```python
from build123d import *

# Parameters (mm, degrees)
F0_W     = 35.2
F0_H     = 35.2
F0_W_2   = 26
F0_H_2   = 26
F0_R     = 11
F0_R_2   = 2.5
F1_DEPTH = 42
F2_DEPTH = 2
F3_DEPTH = 25
F4_R     = 3
F5_D     = 3
F5_DEPTH = 5
F5_TIP   = 0.9012909285


with BuildPart() as f1:
    # F0 (on Top) → F1 (new body)
    with BuildSketch(Plane.XY):
        Rectangle(F0_W, F0_H)
        Rectangle(F0_W_2, F0_H_2, mode=Mode.SUBTRACT)
        Rectangle(F0_W_2, F0_H_2)
        Circle(F0_R, mode=Mode.SUBTRACT)
        Circle(F0_R)
        Circle(F0_R_2, mode=Mode.SUBTRACT)
        Circle(F0_R_2)
    extrude(amount=-F1_DEPTH)

    # F0 (on Top) → F2 (join)
    with BuildSketch(Plane.XY):
        Circle(F0_R)
        Circle(F0_R_2, mode=Mode.SUBTRACT)
    extrude(amount=F2_DEPTH)

    # F0 (on Top) → F3 (join)
    with BuildSketch(Plane.XY):
        Circle(F0_R_2)
    extrude(amount=F3_DEPTH)

    # F4
    f4_edges = [f1.edges().sort_by_distance(p)[0] for p in [
        (17.6, 17.6, -21),
        (17.6, -17.6, -21),
        (-17.6, -17.6, -21),
        (-17.6, 17.6, -21),
    ]]
    fillet(f4_edges, radius=F4_R)

    # F5
    with Locations(Plane.XY):
        with Locations((-13, 13), (13, 13), (13, -13), (-13, -13)):
            Hole(F5_D / 2, depth=F5_DEPTH)
            with Locations((0, 0, -(F5_DEPTH + F5_TIP / 2))):  # 118° drill point
                Cone(0, F5_D / 2, F5_TIP, mode=Mode.SUBTRACT)


solid = f1.part
```
The model under review builds one solid part; all positions refer to its coordinate system, in mm. A direction names the side the tool comes from. Coordinates: 2 decimals unless noted, no trailing zeros. Write each loop counter-clockwise with the first axis right and the second up, starting at its lowest first coordinate (ties: lowest second). Pieces come first, ordered by that corner, then holes. Notation, with made-up numbers: (59.5, -31) -> (83.5, -31) arc R29 ccw to (83.5, -10) -> close; hole circle Ø6 at (8, 43.25). An arc over 180 degrees is marked (long way). One line per item, written item: value. Start each with the question number.
Q1. Clearance check with flat-ended pins moving along their axes: P1, Ø2.5, axis at x = -13, y = -13, coming from the +Z side; P2, Ø8, axis at x = 4, y = -9.5, coming from the +Z side; P3, Ø4, axis at x = -1.5, z = 3.5, coming from the +Y side. State where each tip first meets the part, or that it passes through.
Q2. Add section C-C, the plane x = -9.5. Give the boundary of the cut face in (y, z), then the cut area to 3 significant figures.
Q3. The part is to be moulded in two halves that separate along X. For faces 1 (the face through (-2.38, -10.74, 0.99)), 2 (the face through (-11.5, 13.07, -2.54)), 3 (the face through (14.5, 13.07, -2.54)), 4 (the face through (-16.74, 16.7, -21.29)), say which applies: +X half, -X half, draft (parallel to the pull), parting line (faces both ways), or undercut.
Q4. To check wall thickness, follow probe 1 along Y at (x, z) = (13, -2.85); probe 2 along Z at (x, y) = (-6.5, -14). State the ranges of each line that lie inside material, in increasing order.
Q5. Add section A-A, the plane x = 0. Give the boundary of the cut face in (y, z).
Q6. Add section D-D, the plane y = 7. Give the boundary of the cut face in (x, z).
Q7. For faces 5 (the face through (14.5, -12.93, -2.54)), 6 (the face through (0, 0, -42)), list the 3-axis set-ups (+Z, -Z, +X, -X, +Y, -Y) from which the entire face can be reached by the end or side of a thin tool; tool diameter is ignored.
Response:
1. P1: z = -5.15
1. P2: z = 2
1. P3: y = 11
2. outline: (-17.6, -42) -> (17.6, -42) -> (17.6, 0) -> (5.55, 0) -> (5.55, 2) -> (-5.55, 2) -> (-5.55, 0) -> (-17.6, 0) -> close
2. area: 1,500 mm²
3. face 1: parting line
3. face 2: undercut
3. face 3: undercut
3. face 4: -X half
4. probe 1: -17.6 to -14.5, -11.5 to 11.5, 14.5 to 17.6
4. probe 2: -42 to 0
5. outline: (-17.6, -42) -> (17.6, -42) -> (17.6, 0) -> (11, 0) -> (11, 2) -> (2.5, 2) -> (2.5, 25) -> (-2.5, 25) -> (-2.5, 2) -> (-11, 2) -> (-11, 0) -> (-17.6, 0) -> close
6. outline: (-17.6, -42) -> (17.6, -42) -> (17.6, 0) -> (8.49, 0) -> (8.49, 2) -> (-8.49, 2) -> (-8.49, 0) -> (-17.6, 0) -> close
7. face 5: +Z
7. face 6: -Z, +X, -X, +Y, -Y
